For this review, take the finished solid that the model builds, in its own axes (mm). Give positions to 0.01 mm unless a question says otherwise; leave off trailing zeros. Order: outer loops, then holes, each group sorted by start corner. A loop starts at its lowest first (then second) coordinate and runs counter-clockwise, first axis right, second up. Notation, with made-up numbers: (-27, 87) - (-22, 87) arc R38 cw to (-22, 126) - close; hole circle Ø11 at (-14.75, 40.5). An arc over 180 degrees is marked (long way). One line per item, written item: value.
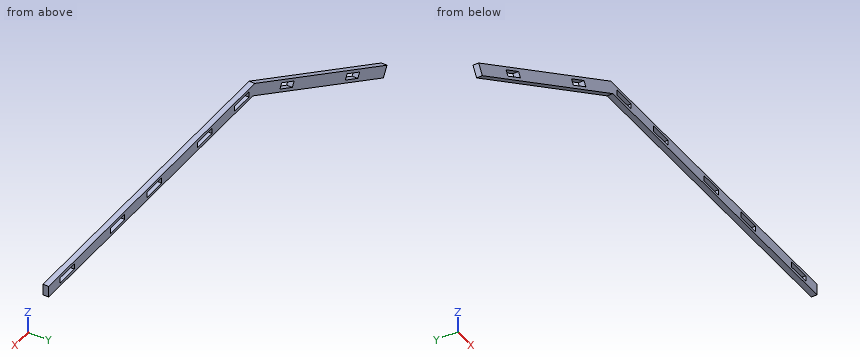
```python
from build123d import *

# Parameters (mm, degrees)
SKETCH4_W           = 25.4
SKETCH4_H           = 6.35
BOSS_EXTRUDE2_DEPTH = 6.35


with BuildPart() as part:
    # Sketch4 → Boss-Extrude2 (new body)
    with BuildSketch(Plane(origin=(0, 0, 0), x_dir=(1, 0, 0), z_dir=(0, 1, 0))):
        Polygon((-596.849633079, 128.276111157), (-590.499633079, 139.274633785), (-360.267413785, 6.35), (0, 6.35), (0, -6.35), (-363.670368529, -6.35), align=None)
        Polygon((-548.51841191, 104.038241814), (-526.521366654, 91.338241814), (-523.346366654, 96.837503128), (-545.34341191, 109.537503128), align=None, mode=Mode.SUBTRACT)
        Polygon((-433.033924315, 37.363241814), (-411.036879059, 24.663241814), (-407.861879059, 30.162503128), (-429.858924315, 42.862503128), align=None, mode=Mode.SUBTRACT)
        with Locations((-340.498292116, 0)):
            Rectangle(SKETCH4_W, SKETCH4_H, mode=Mode.SUBTRACT)
        with Locations((-275.418975234, 0)):
            Rectangle(SKETCH4_W, SKETCH4_H, mode=Mode.SUBTRACT)
        with Locations((-186.518975234, 0)):
            Rectangle(SKETCH4_W, SKETCH4_H, mode=Mode.SUBTRACT)
        with Locations((-121.439658352, 0)):
            Rectangle(SKETCH4_W, SKETCH4_H, mode=Mode.SUBTRACT)
        with Locations((-32.539658352, 0)):
            Rectangle(SKETCH4_W, SKETCH4_H, mode=Mode.SUBTRACT)
    extrude(amount=BOSS_EXTRUDE2_DEPTH)


solid = part.part
```
(1) Take a section at C-C (x = -167). Write out the cut boundary in (y, z).
Answers below:
outline: (0, -6.35) - (6.35, -6.35) - (6.35, 6.35) - (0, 6.35) - close
(2) Wall thickness on line 1 (X direction, y = 5.5, z = -1.5); line 2 (Z direction, x = -351.5, y = 5) (3 decimals); line 3 (Z direction, x = -302, y = 6): over which ranges is each line inside the solid? List them lowest first. Write a range as from..to.
Answers below:
line 1: x = -377.27..-353.2, -327.8..-288.12, -262.72..-199.22, -173.82..-134.14, -108.74..-45.24, -19.84..0
line 2: z = -6.35..-3.175, 3.175..6.35
line 3: z = -6.35..6.35
(3) For P1, Ø2, axis at y = 1, z = -90.5, coming from the -X side; P2, Ø1.9, axis at y = 3.5, z = 1.5, coming from the +X side; P3, Ø1.5, axis at x = -445.5, y = 5.5, coming from the +Z side; P4, Ø3, axis at y = 5.5, z = -30, coming from the +X side, all flat-tipped, find the tip position at first contact; note any pin that passes through.
Answers below:
P1: stops at x = -533.15
P2: stops at x = 0
P3: stops at z = -40.46
P4: stops at x = -398.63
(4) Take a section at B-B (y = 5.25). Give the number of separate pieces and of enclosed holes in the cut face, then the cut area to 3 significant figures.
Answers below:
separate pieces: 1
enclosed holes: 7
area: 6,870 mm^2
(5) Take a section at A-A (x = -338). Write out the cut boundary in (y, z) (3 decimals), then the cut area to 3 significant figures.
Answers below:
outline: (0, -6.35) - (6.35, -6.35) - (6.35, -3.175) - (0, -3.175) - close; (0, 3.175) - (6.35, 3.175) - (6.35, 6.35) - (0, 6.35) - close
area: 40.3 mm^2
(6) Take a section at D-D (z = -58). Write out the cut boundary in (x, y), then the cut area to 3 significant figures.
Answers below:
outline: (-475.13, 0) - (-449.73, 0) - (-449.73, 6.35) - (-475.13, 6.35) - close
area: 161 mm^2
